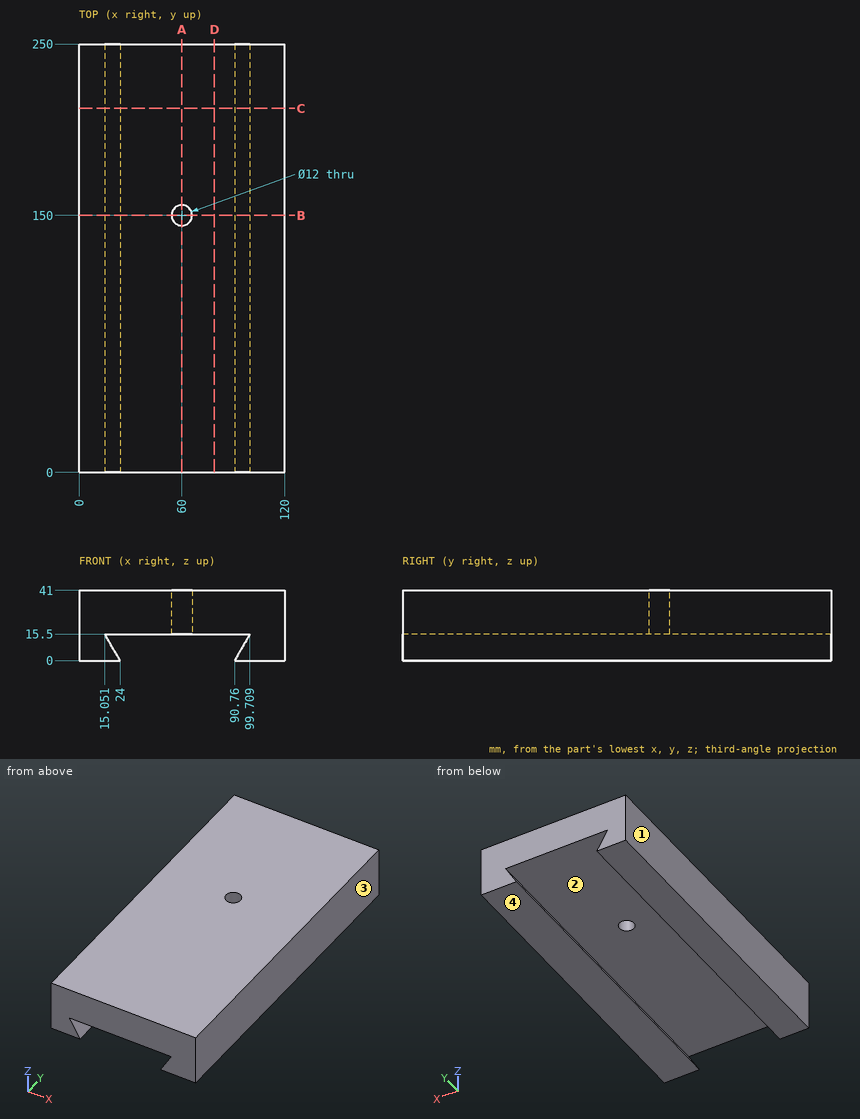
Study the drawing (mm; zero at the part's minimum x, y, z) and answer. Coordinates: 2 decimals unless noted, no trailing zeros. Write each loop counter-clockwise with the first axis right and the second up, starting at its lowest first coordinate (ties: lowest second). Pieces come first, ordered by that corner, then holes. Notation, with made-up numbers: (66.25, 34.25) - (111.25, 34.25) arc R18 ccw to (111.25, 46.25) - close; hole circle Ø6 at (-14.5, 82). An arc over 180 degrees is marked (long way). Return JSON: item names as keys, results as strings. Group by question number.
1. A cutting plane is placed at A-A, the plane x = 60. Determine the outline of the cut face in (y, z), plus the area to 3 significant figures.
2. Determine the mould class of the marked faces 1, 2, 3 and 4 for opening direction X: released by +X, released by -X, zero draft, split by the parting line, or undercut.
3. Given pin 1 (1 mm diameter, centred on x = 70.5, y = 112.5, fed in from -Z), flat-ended and moving along its own axis, determine where the tip first touches the part or whether it passes through.
4. A cutting plane is placed at B-B, the plane y = 150. Determine the outline of the cut face in (x, z), plus the area to 3 significant figures.
5. A cutting plane is placed at D-D, the plane x = 79. Determine the outline of the cut face in (y, z).
6. Straight lines are drawn through the part: L1, parallel to Y at x = 60, z = 25; L2, parallel to Z at x = 75.5, y = 30; L3, parallel to X at y = 49.5, z = 12. For each, find the intervals that lie inside material, in ascending order.
7. A cutting plane is placed at C-C, the plane y = 212.5. Determine the outline of the cut face in (x, z).
Ans:
{
 "1": {"outline": "(0, 15.5) - (144, 15.5) - (144, 41) - (0, 41) - close; (156, 15.5) - (250, 15.5) - (250, 41) - (156, 41) - close", "area": "6,070 mm²"},
 "2": {"face 1": "released by -X", "face 2": "undercut", "face 3": "released by +X", "face 4": "zero draft"},
 "3": {"pin 1": "z = 15.5"},
 "4": {"outline": "(0, 0) - (24, 0) - (15.05, 15.5) - (54, 15.5) - (54, 41) - (0, 41) - close; (66, 15.5) - (99.71, 15.5) - (90.76, 0) - (120, 0) - (120, 41) - (66, 41) - close", "area": "3,440 mm²"},
 "5": {"outline": "(0, 15.5) - (250, 15.5) - (250, 41) - (0, 41) - close"},
 "6": {"L1": "0 to 144, 156 to 250", "L2": "15.5 to 41", "L3": "0 to 17.07, 97.69 to 120"},
 "7": {"outline": "(0, 0) - (24, 0) - (15.05, 15.5) - (99.71, 15.5) - (90.76, 0) - (120, 0) - (120, 41) - (0, 41) - close"}
}
